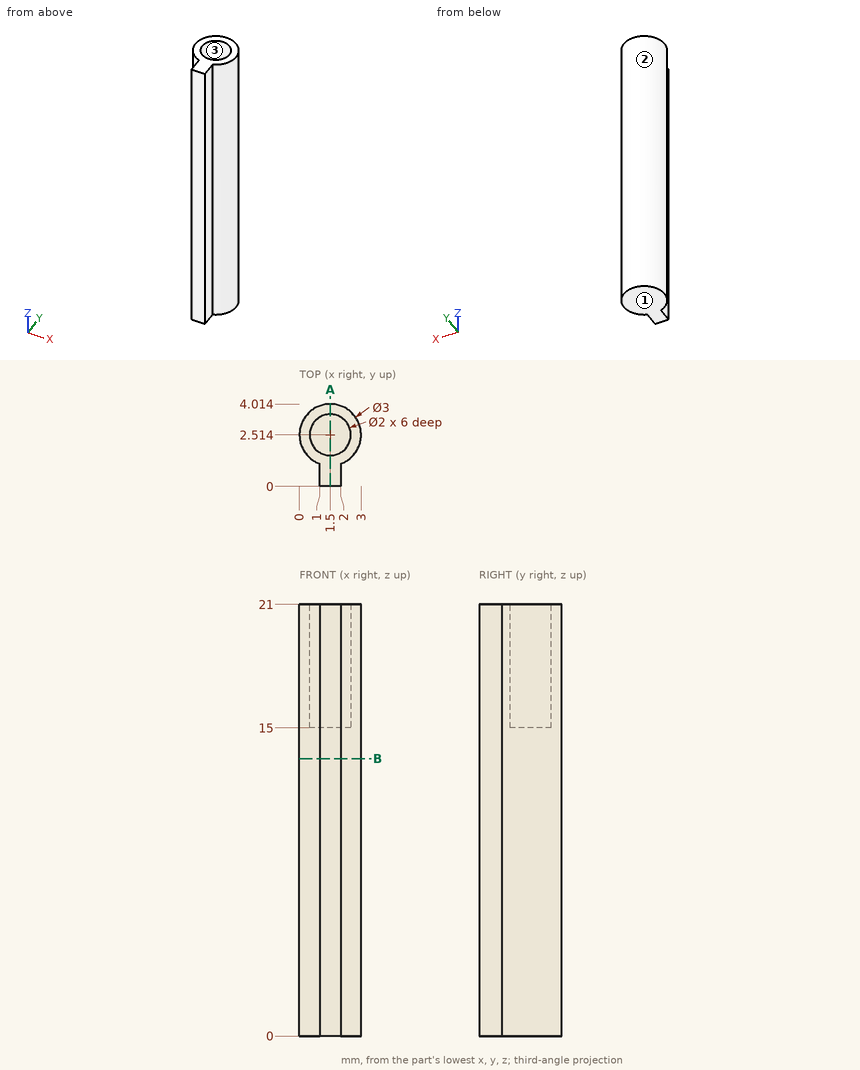
Can you work these out from the drawing? Everything is in mm from the part's minimum corner. Round coordinates to 2 decimals unless told otherwise and drop trailing zeros. Loops run counter-clockwise (first coordinate to the right, second up) from the corner with the lowest first, then second, coordinate; pieces in that order, holes last.
1. If we section it at B-B on z = 13.5: Write out the boundary of the cut face in (x, y).
Answer list:
outline: (1, 0) - (2, 0) - (2, 1.1) arc R1.5 ccw (long way) to (1, 1.1) - close
2. We'd pull the mould along X, two halves only. Please class the marked faces 1, 2 and 3: +X half, -X half, draft (parallel to the pull), parting line (faces both ways), or undercut.
Answer list:
face 1: draft
face 2: parting line
face 3: undercut
3. If we section it at A-A on x = 1.5: Write out the boundary of the cut face in (y, z), plus the area to 3 significant figures.
Answer list:
outline: (0, 0) - (4.01, 0) - (4.01, 21) - (3.51, 21) - (3.51, 15) - (1.51, 15) - (1.51, 21) - (0, 21) - close
area: 72.3 mm2
4. If I drill on line 1 along Y through (x, z) = (1.5, 18.2); line 2 along Z through (x, y) = (2.4, 2.7); line 3 along X through (y, z) = (3.05, 17) (1 decimal), over which ranges is the centre line in solid material (lowest first)?
Answer list:
line 1: y = 0 to 1.51, 3.51 to 4.01
line 2: z = 0 to 15
line 3: x = 0.1 to 0.7, 2.3 to 2.9
5. For P1, Ø1.2, axis at y = 1, z = 14.5, coming from the -X side; P2, Ø0.9, axis at y = 0.5, z = 14.5, coming from the +X side; P3, Ø1, axis at x = 2.5, z = 4.5, coming from the +Y side, each with a flat end and sliding along its axis, tell me the tip position at first contact or that it passes through.
Answer list:
P1: stops at x = 0.31
P2: stops at x = 2
P3: stops at y = 3.93
